Here's how the part is built. I have some questions about the finished solid (model axes, mm). Give positions to 0.01 mm unless a question says otherwise; leave off trailing zeros. Loops run counter-clockwise (first coordinate to the right, second up) from the corner with the lowest first, then second, coordinate; pieces in that order, holes last. Notation, with made-up numbers: (-31.5, -36.75) - (18.5, -36.75) arc R10 ccw to (18.5, -29.75) - close; hole circle Ø9 at (21, -12). An arc over 180 degrees is marked (long way). Return JSON: item names as keys, results as strings. Group by question number.
(1) If we section it at C-C (z = 5): Please give me the cut outline in (x, y).
(2) If we section it at D-D (x = -47): Please give me the cut outline in (y, z), then the cut area to 3 significant figures.
(3) If we section it at A-A (x = 47): Please give me the cut outline in (y, z), then the cut area to 3 significant figures.
(4) If we section it at B-B (y = 22): Please give me the cut outline in (x, z), then the cut area to 3 significant figures.
(5) For P1, Ø3, axis at y = -4, z = 1.5, coming from the -X side, with a flat end and sliding along its axis, tell me the tip position at first contact or that it passes through.
(6) I need wall thicknesses on probe 1 along Y at (x, z) = (-47, 4.5); probe 2 along Y at (x, z) = (47, 1.5); probe 3 along Y at (x, z) = (38, 2.5). Which ranges of each line are inside material? Lowest first, please. Write a range as [from, to].
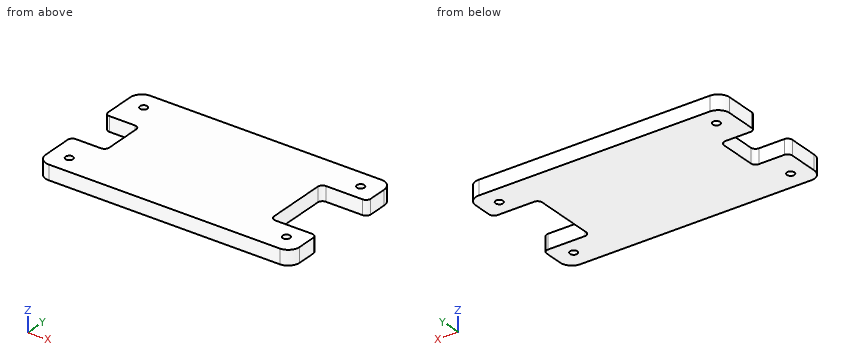
```python
from build123d import *

# Parameters (mm, degrees)
F0_R     = 1.6
F1_DEPTH = 6.35
F2_R     = 5
F3_R     = 2


with BuildPart() as f1:
    # F0 (on Top) → F1 (new body)
    with BuildSketch(Plane.XY):
        Polygon((55, 30), (-55, 30), (-55, 10), (-40, 10), (-40, -10), (-55, -10), (-55, -30), (55, -30), (55, -15), (35, -15), (35, 15), (55, 15), align=None)
        with Locations((-47, -22)):
            Circle(F0_R, mode=Mode.SUBTRACT)
        with Locations((47, -22)):
            Circle(F0_R, mode=Mode.SUBTRACT)
        with Locations((-47, 22)):
            Circle(F0_R, mode=Mode.SUBTRACT)
        with Locations((47, 22)):
            Circle(F0_R, mode=Mode.SUBTRACT)
    extrude(amount=F1_DEPTH)

    # F2
    f2_edges = [f1.edges().sort_by_distance(p)[0] for p in [
        (-55, 30, 3.175),
        (55, 30, 3.175),
        (55, -30, 3.175),
        (-55, -30, 3.175),
    ]]
    fillet(f2_edges, radius=F2_R)

    # F3
    f3_edges = [f1.edges().sort_by_distance(p)[0] for p in [
        (-55, -10, 3.175),
        (-40, -10, 3.175),
        (-55, 10, 3.175),
        (-40, 10, 3.175),
        (35, -15, 3.175),
        (55, -15, 3.175),
        (55, 15, 3.175),
        (35, 15, 3.175),
    ]]
    fillet(f3_edges, radius=F3_R)


solid = f1.part
```
Values:
{
 "1": {"outline": "(-55, -25) arc R5 ccw to (-50, -30) - (50, -30) arc R5 ccw to (55, -25) - (55, -17) arc R2 ccw to (53, -15) - (37, -15) arc R2 cw to (35, -13) - (35, 13) arc R2 cw to (37, 15) - (53, 15) arc R2 ccw to (55, 17) - (55, 25) arc R5 ccw to (50, 30) - (-50, 30) arc R5 ccw to (-55, 25) - (-55, 12) arc R2 ccw to (-53, 10) - (-42, 10) arc R2 cw to (-40, 8) - (-40, -8) arc R2 cw to (-42, -10) - (-53, -10) arc R2 ccw to (-55, -12) - close; hole circle Ø3.2 at (-47, -22); hole circle Ø3.2 at (-47, 22); hole circle Ø3.2 at (47, -22); hole circle Ø3.2 at (47, 22)"},
 "2": {"outline": "(-30, 0) - (-23.6, 0) - (-23.6, 6.35) - (-30, 6.35) - close; (-20.4, 0) - (-10, 0) - (-10, 6.35) - (-20.4, 6.35) - close; (10, 0) - (20.4, 0) - (20.4, 6.35) - (10, 6.35) - close; (23.6, 0) - (30, 0) - (30, 6.35) - (23.6, 6.35) - close", "area": "213 mm2"},
 "3": {"outline": "(-30, 0) - (-23.6, 0) - (-23.6, 6.35) - (-30, 6.35) - close; (-20.4, 0) - (-15, 0) - (-15, 6.35) - (-20.4, 6.35) - close; (15, 0) - (20.4, 0) - (20.4, 6.35) - (15, 6.35) - close; (23.6, 0) - (30, 0) - (30, 6.35) - (23.6, 6.35) - close", "area": "150 mm2"},
 "4": {"outline": "(-55, 0) - (-48.6, 0) - (-48.6, 6.35) - (-55, 6.35) - close; (-45.4, 0) - (45.4, 0) - (45.4, 6.35) - (-45.4, 6.35) - close; (48.6, 0) - (55, 0) - (55, 6.35) - (48.6, 6.35) - close", "area": "658 mm2"},
 "5": {"P1": "x = -40"},
 "6": {"probe 1": "[-30, -23.6], [-20.4, -10], [10, 20.4], [23.6, 30]", "probe 2": "[-30, -23.6], [-20.4, -15], [15, 20.4], [23.6, 30]", "probe 3": "[-30, -15], [15, 30]"}
}
